Here's how the part is built. I have some questions about the finished solid (model axes, mm). Give positions to 0.01 mm unless a question says otherwise; leave off trailing zeros. Write each loop counter-clockwise with the first axis right and the second up, starting at its lowest first coordinate (ties: lowest second). Pieces come first, ordered by that corner, then holes. Notation, with made-up numbers: M 10,-32 L 15,-32 A5 cw 15,-24 Z; hole C -18,62 d4. An arc over 180 degrees is marked long. Answer as CSV lines item,"result". Start each with the question number.
Q1. For pin 1 (6 mm diameter, centred on y = 119.5, z = 7.5, fed in from -X); pin 2 (3 mm diameter, centred on y = 145, z = 4.5, fed in from -X), each with a flat end and sliding along its axis, tell me the tip position at first contact or that it passes through.
Q2. Suppose I cut it at C-C (z = 7.75). Write out the boundary of the cut face in (x, y).
Q3. If I drill on line 1 along X through (y, z) = (166.5, 5); line 2 along Y through (x, z) = (-8.5, 2); line 3 along X through (y, z) = (138, 1.5), over which ranges is the centre line in solid material (lowest first)?
Q4. Suppose I cut it at B-B (y = 162). Write out the boundary of the cut face in (x, z), then the cut area to 3 significant figures.
Q5. Suppose I cut it at A-A (x = 20.5). Write out the boundary of the cut face in (y, z).
```python
from build123d import *

# Parameters (mm, degrees)
F0_W        = 121.859960258
F0_H        = 246.6522753239
F1_DEPTH    = 10
F2_SIZE2    = 5
F2_SIZE     = 12
F3_SIZE2    = 5
F3_SIZE     = 12
F4_T1_DEPTH = 172.0821922482
F5_T1_DEPTH = 291.8745073141
F6_SIZE2    = 5
F6_SIZE     = 12
F7_SIZE2    = 5
F7_SIZE     = 12


# Not quite as in the source:
# - a fillet or chamfer that OpenCascade refuses, or shapes differently, is made with other operations: its cross-section is extruded or revolved along the edge and cut away or added


with BuildPart() as f1:
    # F0 (on Top) → F1 (new body)
    with BuildSketch(Plane.XY):
        with Locations((24.3507884443, 90.4376059771)):
            Rectangle(F0_W, F0_H)
    extrude(amount=F1_DEPTH)

    # F2
    f2_edges = [f1.edges().sort_by_distance(p)[0] for p in [
        (85.280769, 90.437606, 10),
    ]]
    f2_side = f1.faces().sort_by_distance((24.350788, 90.437606, 10))[0]
    chamfer(f2_edges, length=F2_SIZE, length2=F2_SIZE2, reference=f2_side)

    # F3
    f3_edges = [f1.edges().sort_by_distance(p)[0] for p in [
        (18.350788, -32.888532, 10),
    ]]
    f3_side = f1.faces().sort_by_distance((18.350788, 90.437606, 10))[0]
    chamfer(f3_edges, length=F3_SIZE, length2=F3_SIZE2, reference=f3_side)

    # F4: chamfer of 12 x 5 on 1 edges, made by hand

    # F4_s2 → F4_t1 (cut)
    with BuildSketch(Plane.YZ.offset(-67.6903076798)):
        Polygon((208.763743639, 10), (213.763743639, -2), (213.763743639, 10), align=None)
    extrude(amount=F4_T1_DEPTH, mode=Mode.SUBTRACT)

    # F5: chamfer of 12 x 5 on 1 edges, made by hand

    # F5_s2 → F5_t1 (cut)
    with BuildSketch(Plane.XZ.offset(-239.8748596341)):
        Polygon((-36.5791916847, -2), (-31.5791916847, 10), (-36.5791916847, 10), align=None)
    extrude(amount=F5_T1_DEPTH, mode=Mode.SUBTRACT)

    # F6
    f6_edges = [f1.edges().sort_by_distance(p)[0] for p in [
        (-31.579192, 93.937606, 10),
    ]]
    f6_side = f1.faces().sort_by_distance((20.850788, 93.937606, 10))[0]
    chamfer(f6_edges, length=F6_SIZE, length2=F6_SIZE2, reference=f6_side)

    # F7
    f7_edges = [f1.edges().sort_by_distance(p)[0] for p in [
        (26.850788, 208.763744, 10),
    ]]
    f7_side = f1.faces().sort_by_distance((26.850788, 93.937606, 10))[0]
    chamfer(f7_edges, length=F7_SIZE, length2=F7_SIZE2, reference=f7_side)


solid = f1.part
```
Resolved:
1,pin 1,"x = -33.87"
1,pin 2,"x = -34.5"
2,outline,"M -26.37,-26.29 L 78.68,-26.29 L 78.68,203.55 L -26.37,203.55 Z"
3,line 1,"-33.66 to 85.28"
3,line 2,"-32.89 to 212.1"
3,line 3,"-35.12 to 85.28"
4,outline,"M -35.75,0 L 85.28,0 L 85.28,5 L 73.28,10 L -19.58,10 L -33.5,5.38 Z"
4,area,"1,130 mm^2"
5,outline,"M -32.89,0 L 212.93,0 L 210.69,5.38 L 196.76,10 L -20.89,10 L -32.89,5 Z"
